Work out the finished part from the listing and answer in its coordinate system (mm). A direction names the side the tool comes from. Round coordinates to 2 decimals unless told otherwise and drop trailing zeros. Order: outer loops, then holes, each group sorted by start corner. A loop starts at its lowest first (then second) coordinate and runs counter-clockwise, first axis right, second up. Notation, with made-up numbers: (88, -29) -> (115, -29) arc R22 cw to (115, -23) -> close; hole circle Ø7 at (43.5, 61.5). An arc over 180 degrees is marked (long way). Use one line per item in the form item = value.
```python
from build123d import *

# Parameters (mm, degrees)
BOSS_EXTRU_1_DEPTH       = 13
COQUE1_T                 = -5
COQUE1_THICKNESS_2_DEPTH = 2
ESQUISSE2_R              = 2.5
ENL_V_MAT_EXTRU_1_DEPTH  = 5
ESQUISSE3_R              = 2.5
ENL_V_MAT_EXTRU_2_DEPTH  = 5
BOSS_EXTRU_2_DEPTH       = 10


with BuildPart() as part:
    # Esquisse1 → Boss.-Extru.1 (new body)
    with BuildSketch(Plane.XY):
        with BuildLine():
            Line((-20.881563692, 33.728448276), (44.118436308, 33.728448276))
            ThreePointArc((44.118436308, 33.728448276), (51.18950412, 30.799516088), (54.118436308, 23.728448276))
            Line((54.118436308, 23.728448276), (54.118436308, -41.271551724))
            Line((54.118436308, -41.271551724), (-20.881563692, -41.271551724))
            Line((-20.881563692, -41.271551724), (-20.881563692, 33.728448276))
        make_face()
    extrude(amount=BOSS_EXTRU_1_DEPTH)

    # Coque1
    coque1_openings = [part.faces().sort_by_distance(p)[0] for p in [
        (16.483374946, -3.906613086, 13),
    ]]
    offset(amount=COQUE1_T, openings=coque1_openings, kind=Kind.INTERSECTION)

    # Coque1 thickness 2 face (on inner face of the shell) → Coque1 thickness 2 (cut)
    with BuildSketch(Plane(origin=(16.578534255, -3.811453777, 5), x_dir=(-1, 0, 0), z_dir=(0, 0, -1))):
        with BuildLine():
            Line((-27.539902053, 32.539902053), (32.460097947, 32.539902053))
            Line((32.460097947, 32.539902053), (32.460097947, -32.460097947))
            Line((32.460097947, -32.460097947), (-32.539902053, -32.460097947))
            Line((-32.539902053, -32.460097947), (-32.539902053, 27.539902053))
            ThreePointArc((-32.539902053, 27.539902053), (-31.075435959, 31.075435959), (-27.539902053, 32.539902053))
        make_face()
    extrude(amount=COQUE1_THICKNESS_2_DEPTH, mode=Mode.SUBTRACT)

    # Esquisse2 → Enlèv. mat.-Extru.1 (cut)
    with BuildSketch(Plane.ZY.offset(20.881563692)):
        with Locations(Location((8, -16.271551724, 0), (0, 0, 270))):
            Circle(ESQUISSE2_R)
        with Locations(Location((8, 8.728448276, 0), (0, 0, 270))):
            Circle(ESQUISSE2_R)
    extrude(amount=-ENL_V_MAT_EXTRU_1_DEPTH, mode=Mode.SUBTRACT)

    # Esquisse3 → Enlèv. mat.-Extru.2 (cut)
    with BuildSketch(Plane.XZ.offset(41.271551724)):
        with Locations(Location((4.118436308, 8, 0), (0, 0, 270))):
            Circle(ESQUISSE3_R)
        with Locations(Location((29.118436308, 8, 0), (0, 0, 270))):
            Circle(ESQUISSE3_R)
    extrude(amount=-ENL_V_MAT_EXTRU_2_DEPTH, mode=Mode.SUBTRACT)

    # Esquisse4 → Boss.-Extru.2 (add)
    with BuildSketch(Plane.XY.offset(3)):
        Polygon((-15.881563692, -26.271551724), (-5.881563692, -36.271551724), (-15.881563692, -36.271551724), align=None)
    extrude(amount=BOSS_EXTRU_2_DEPTH)


solid = part.part
```
Item 1: Determine the mould class of faces 5 (the cylindrical face through (-18.417, -14.288, 6.479)), 6 (the flat face through (17, -41.272, 6)), 7 (the flat face through (17, -3, 0)), 8 (the flat face through (16, -3, 3)) for opening direction Z: released by +Z, released by -Z, zero draft, split by the parting line, or undercut.
Findings:
face_5 = undercut
face_6 = zero draft
face_7 = released by -Z
face_8 = released by +Z
Item 2: For faces 1 (the cylindrical face through (4.2, -38.8, 10.5)), 2 (the cylindrical face through (-18.417, 7.575, 5.782)), 3 (the flat face through (49.118, -6, 8)), 4 (the cylindrical face through (51.11, 30.88, 6.41)), determine the directions among +Z, -Z, +X, -X, +Y, -Y from which every point of the face is accessible in a straight line to the end or side of a thin tool.
Findings:
face_1 = -Y
face_2 = -X
face_3 = +Z
face_4 = +Z, -Z, +X, +Y
Item 3: The part is cut by section B-B, the plane x = 36. Give the vertices of the cut face in (y, z), and give its area (3 significant figures).
Findings:
outline = (-41.27, 0) -> (33.73, 0) -> (33.73, 13) -> (28.73, 13) -> (28.73, 3) -> (-36.27, 3) -> (-36.27, 13) -> (-41.27, 13) -> close
area = 325 mm^2
Item 4: Flat-ended cylindrical pins translate along their axes: P1, Ø1.5, axis at x = 46, z = 4.5, coming from the +Y side; P2, Ø4.5, axis at x = 4.12, z = 8, coming from the -Y side. Find the tip coordinate at first contact, or state that the pin passes through.
Findings:
P1 = 33.66
P2 = 28.73
Item 5: Consider line 1 along Y through (x, z) = (30, 5.5); line 2 along X through (y, z) = (22, 4.5); line 3 along Z through (x, y) = (-10.5, 3). Determine where each line is inside the solid, lowest interval first.
Findings:
line_1 = -41.27 to -36.27, 28.73 to 33.73
line_2 = -20.88 to -15.88, 49.12 to 54.12
line_3 = 0 to 3
Item 6: The part is cut by section A-A, the plane z = 8. Give the vertices of the cut face in (x, y).
Findings:
outline = (-20.88, -41.27) -> (1.62, -41.27) -> (1.62, -36.27) -> (-5.88, -36.27) -> (-15.88, -26.27) -> (-15.88, -18.77) -> (-20.88, -18.77) -> close; (-20.88, -13.77) -> (-15.88, -13.77) -> (-15.88, 6.23) -> (-20.88, 6.23) -> close; (-20.88, 11.23) -> (-15.88, 11.23) -> (-15.88, 28.73) -> (44.12, 28.73) arc R5 cw to (49.12, 23.73) -> (49.12, -36.27) -> (31.62, -36.27) -> (31.62, -41.27) -> (54.12, -41.27) -> (54.12, 23.73) arc R10 ccw to (44.12, 33.73) -> (-20.88, 33.73) -> close; (6.62, -41.27) -> (26.62, -41.27) -> (26.62, -36.27) -> (6.62, -36.27) -> close
